```python
from build123d import *

# Parameters (mm, degrees)
F0_R     = 15.875
F0_R_2   = 9.525
F1_DEPTH = 25.4
F2_DEPTH = 25.4
F3_DEPTH = 12.7
F4_R     = 6.35


with BuildPart() as f1:
    # F0 (on Top) → F1 (new body)
    with BuildSketch(Plane.XY):
        with BuildLine():
            ThreePointArc((7.9032867525, -27.4603110599), (22.829444189, -17.1856656264), (28.575, 0))
            ThreePointArc((28.575, 0), (22.829444189, 17.1856656264), (7.9032867525, 27.4603110599))
            ThreePointArc((7.9032867525, 27.4603110599), (-28.575, 0), (7.9032867525, -27.4603110599))
        make_face()
        Circle(F0_R, mode=Mode.SUBTRACT)
        with BuildLine():
            ThreePointArc((7.9032867525, 27.4603110599), (22.829444189, 17.1856656264), (28.575, 0))
            ThreePointArc((28.575, 0), (22.829444189, -17.1856656264), (7.9032867525, -27.4603110599))
            Line((7.9032867525, -27.4603110599), (50.8, -19.05))
            ThreePointArc((50.8, -19.05), (31.75, 0), (50.8, 19.05))
            Line((50.8, 19.05), (7.9032867525, 27.4603110599))
        make_face()
        with BuildLine():
            ThreePointArc((69.85, 0), (64.2703841816, 13.4703841816), (50.8, 19.05))
            ThreePointArc((50.8, 19.05), (31.75, 0), (50.8, -19.05))
            ThreePointArc((50.8, -19.05), (64.2703841816, -13.4703841816), (69.85, 0))
        make_face()
        with Locations((50.8, 0)):
            Circle(F0_R_2, mode=Mode.SUBTRACT)
    extrude(amount=-F1_DEPTH)

    # F0 (on Top) → F2 (join)
    with BuildSketch(Plane.XY):
        with BuildLine():
            ThreePointArc((7.9032867525, -27.4603110599), (22.829444189, -17.1856656264), (28.575, 0))
            ThreePointArc((28.575, 0), (22.829444189, 17.1856656264), (7.9032867525, 27.4603110599))
            ThreePointArc((7.9032867525, 27.4603110599), (-28.575, 0), (7.9032867525, -27.4603110599))
        make_face()
        Circle(F0_R, mode=Mode.SUBTRACT)
    extrude(amount=F2_DEPTH)

    # F0 (on Top) → F3 (cut)
    with BuildSketch(Plane.XY):
        with BuildLine():
            ThreePointArc((69.85, 0), (64.2703841816, 13.4703841816), (50.8, 19.05))
            ThreePointArc((50.8, 19.05), (31.75, 0), (50.8, -19.05))
            ThreePointArc((50.8, -19.05), (64.2703841816, -13.4703841816), (69.85, 0))
        make_face()
        with Locations((50.8, 0)):
            Circle(F0_R_2, mode=Mode.SUBTRACT)
    extrude(amount=-F3_DEPTH, mode=Mode.SUBTRACT)

    # F4
    f4_edges = [f1.edges().sort_by_distance(p)[0] for p in [
        (50.8, 19.05, -6.35),
        (50.8, -19.05, -6.35),
    ]]
    fillet(f4_edges, radius=F4_R)


solid = f1.part
```
Geometry check sheet. Reference: the model listing, model coordinates, mm. A direction names the side the tool comes from. Round coordinates to 2 decimals unless told otherwise and drop trailing zeros. Order: outer loops, then holes, each group sorted by start corner. A loop starts at its lowest first (then second) coordinate and runs counter-clockwise, first axis right, second up. Notation, with made-up numbers: (-30, 19) - (17, 19) arc R9 cw to (17, 24) - close; hole circle Ø4 at (15.25, -8). An arc over 180 degrees is marked (long way). Use a Markdown table: item, result. Add a question column.
(1) Depth check by flat-ended pin: pin 1 (19 mm diameter, centred on x = 47.5, y = 8.5, fed in from +Z); pin 2 (10 mm diameter, centred on y = 10.5, z = 11.5, fed in from -X); pin 3 (2 mm diameter, centred on x = -17.5, z = 10.5, fed in from -Y). Enter the tip coordinate at first touch or a pass-through.
(2) Sectioned sample at D-D, the plane x = 13. Enter the section's corners in (y, z), and give its area (3 significant figures).
(3) Release check for a two-part mould opening along Y. For faces 3 (the cylindrical face through (69.845, -0.419, -18.961)), 4 (the flat face through (24.285, -24.249, -15.344)), 5 (the cylindrical face through (37.412, -18.403, -6.439)), 6 (the cylindrical face through (-3.441, -15.497, -0.356)) record: pulls with the +Y half, pulls with the -Y half, needs draft (parallel to the pull), parting line crosses it, or undercut.
(4) Sectioned sample at B-B, the plane z = -21. Enter the section's corners in (x, y) (3 decimals), and give its area (3 significant figures).
(5) Material ranges on line 1 along X through (y, z) = (-2, -15); line 2 along Y through (x, z) = (50.8, -21) (3 decimals); line 3 along Y through (x, z) = (0, 15) (3 decimals), recorded low to high. Write a range as [from, to].
(6) Tool access check on faces 1 (the flat face through (20, 0, -25.4)), 2 (the flat face through (29, -2, 0)). Record the directions out of +Z, -Z, +X, -X, +Y, -Y that give a thin tool (end or side, any length) a straight path to the whole face; none if there is none.
(7) Sectioned sample at A-A, the plane x = 0. Enter the section's corners in (y, z) (3 decimals), and give its area (3 significant figures).
(8) Sectioned sample at C-C, the plane y = -14. Enter the section's corners in (x, z), and give its area (3 significant figures).
Answers below:
| question | item | result |
|---|---|---|
| 1 | pin 1 | z = -12.7 |
| 1 | pin 2 | x = -28.04 |
| 1 | pin 3 | y = -23.33 |
| 2 | outline | (-26.46, -25.4) - (-9.11, -25.4) - (-9.11, 25.4) - (-25.45, 25.4) - (-25.45, 0) - (-26.46, 0) - close; (9.11, -25.4) - (26.46, -25.4) - (26.46, 0) - (25.45, 0) - (25.45, 25.4) - (9.11, 25.4) - close |
| 2 | area | 1,710 mm² |
| 3 | face 3 | parting line crosses it |
| 3 | face 4 | pulls with the -Y half |
| 3 | face 5 | undercut |
| 3 | face 6 | undercut |
| 4 | outline | (7.903, -27.46) - (50.8, -19.05) arc R19.05 ccw to (50.8, 19.05) - (7.903, 27.46) arc R28.575 ccw (long way) to start; hole circle Ø31.75 at (0, 0); hole circle Ø19.05 at (50.8, 0) |
| 4 | area | 3,220 mm² |
| 5 | line 1 | [-28.5, -15.75], [15.75, 41.49], [60.11, 69.74] |
| 5 | line 2 | [-19.05, -9.525], [9.525, 19.05] |
| 5 | line 3 | [-28.575, -15.875], [15.875, 28.575] |
| 6 | face 1 | -Z, +X, -X, +Y, -Y |
| 6 | face 2 | +Z, +X |
| 7 | outline | (-28.575, -25.4) - (-15.875, -25.4) - (-15.875, 25.4) - (-28.575, 25.4) - close; (15.875, -25.4) - (28.575, -25.4) - (28.575, 25.4) - (15.875, 25.4) - close |
| 7 | area | 1,290 mm² |
| 8 | outline | (-24.91, -25.4) - (-7.48, -25.4) - (-7.48, 25.4) - (-24.91, 25.4) - close; (7.48, -25.4) - (63.72, -25.4) - (63.72, -12.7) - (37.28, -12.7) - (37.28, 0) - (24.91, 0) - (24.91, 25.4) - (7.48, 25.4) - close |
| 8 | area | 2,420 mm² |
